Answer from the drawing. Dimensions are ordinates in mm from the lowest x, y and z of the part. A direction names the side the tool comes from. Give positions to 0.01 mm unless a question says otherwise; leave off trailing zeros. Loops run counter-clockwise (first coordinate to the right, second up) from the corner with the lowest first, then second, coordinate; pieces in that order, holes last. Notation, with made-up numbers: M -38,42 L -9,42 A16 cw -9,70 Z; hole C 21.25,6 d2. An arc over 180 degrees is marked long. Use a Markdown table: item, result.
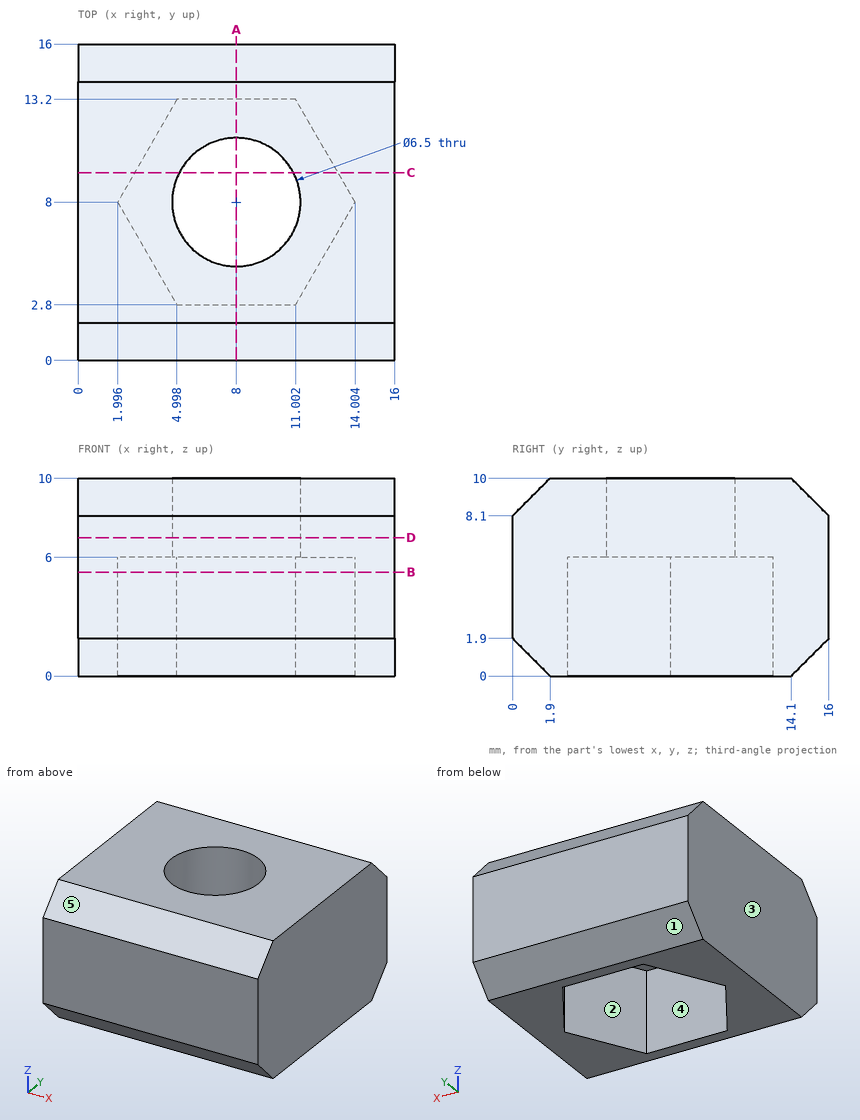
(1) The mould has two halves that part along X. Classify the marked faces 1, 2 and 3: released by +X, released by -X, zero draft, split by the parting line, or undercut.
Entries:
| item | result |
|---|---|
| face 1 | zero draft |
| face 2 | undercut |
| face 3 | released by -X |
(2) A cutting plane is placed at C-C (y = 9.5). Write down the section's boundary in (x, z).
Entries:
| item | result |
|---|---|
| outline | M 0,0 L 2.86,0 L 2.86,6 L 5.12,6 L 5.12,10 L 0,10 Z; M 10.88,6 L 13.14,6 L 13.14,0 L 16,0 L 16,10 L 10.88,10 Z |
(3) A cutting plane is placed at D-D (z = 7). Write down the section's boundary in (x, y).
Entries:
| item | result |
|---|---|
| outline | M 0,0 L 16,0 L 16,16 L 0,16 Z; hole C 8,8 d6.5 |
(4) Consider probe 1 along Y at (x, z) = (10.5, 5); probe 2 along Y at (x, z) = (8, 7.3); probe 3 along Z at (x, y) = (11.5, 6). Determine where each line is inside the solid, lowest interval first. Write a range as [from, to].
Entries:
| item | result |
|---|---|
| probe 1 | y = [0, 2.8], [13.2, 16] |
| probe 2 | y = [0, 4.75], [11.25, 16] |
| probe 3 | z = [6, 10] |
(5) A cutting plane is placed at A-A (x = 8). Write down the section's boundary in (y, z).
Entries:
| item | result |
|---|---|
| outline | M 0,1.9 L 1.9,0 L 2.8,0 L 2.8,6 L 4.75,6 L 4.75,10 L 1.9,10 L 0,8.1 Z; M 11.25,6 L 13.2,6 L 13.2,0 L 14.1,0 L 16,1.9 L 16,8.1 L 14.1,10 L 11.25,10 Z |
(6) Which of the six approach directions +Z, -Z, +X, -X, +Y, -Y give full straight-line access (tool end or side, diameter ignored) to the marked faces 4 and 5?
Entries:
| item | result |
|---|---|
| face 4 | -Z |
| face 5 | +Z, +X, -X, -Y |
(7) A cutting plane is placed at B-B (z = 5.25). Write down the section's boundary in (x, y) (1 decimal).
Entries:
| item | result |
|---|---|
| outline | M 0,0 L 16,0 L 16,16 L 0,16 Z; hole M 2,8 L 5,2.8 L 11,2.8 L 14,8 L 11,13.2 L 5,13.2 Z |
